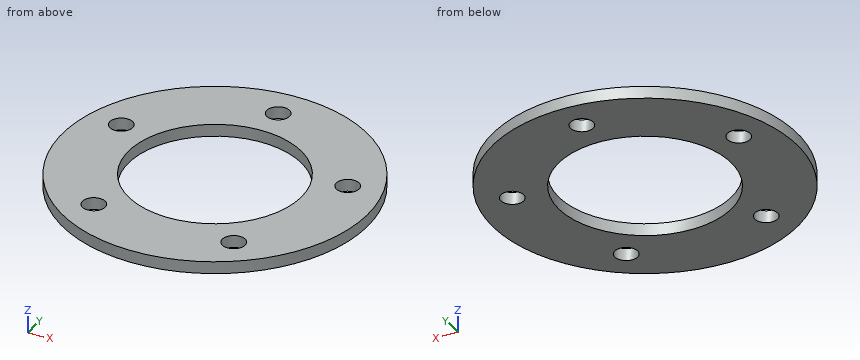
```python
from build123d import *

# Parameters (mm, degrees)
F0_R     = 38.1
F0_R_2   = 2.8575
F0_R_3   = 21.59
F1_DEPTH = 3.048


with BuildPart() as f1:
    # F0 (on Top) → F1 (new body)
    with BuildSketch(Plane.XY):
        Circle(F0_R)
        with Locations((-17.542451, -24.145112)):
            Circle(F0_R_2, mode=Mode.SUBTRACT)
        with Locations((17.542451, -24.145112)):
            Circle(F0_R_2, mode=Mode.SUBTRACT)
        with Locations((-28.384282, 9.222612)):
            Circle(F0_R_2, mode=Mode.SUBTRACT)
        Circle(F0_R_3, mode=Mode.SUBTRACT)
        with Locations((28.384282, 9.222612)):
            Circle(F0_R_2, mode=Mode.SUBTRACT)
        with Locations((0, 29.845)):
            Circle(F0_R_2, mode=Mode.SUBTRACT)
    extrude(amount=F1_DEPTH)


solid = f1.part
```
Read the model definition and answer for the solid it produces. Units are mm, in the model's axes. Coordinates: 2 decimals unless noted, no trailing zeros. Order: outer loops, then holes, each group sorted by start corner. A loop starts at its lowest first (then second) coordinate and runs counter-clockwise, first axis right, second up. Notation, with made-up numbers: (46.25, 30.25) - (72.25, 30.25) arc R13 cw to (72.25, 55.25) - close; hole circle Ø2 at (4, 56.25). An arc over 180 degrees is marked (long way). Answer as a JSON object with one key per item and string values. Group by question number.
Item 1: Consider probe 1 along Y at (x, z) = (0, 1.8); probe 2 along Y at (x, z) = (18.5, 2); probe 3 along X at (y, z) = (-25, 1.9). Determine where each line is inside the solid, lowest interval first. Write a range as from..to.
Item 2: Flat-ended cylindrical pins translate along their axes: P1, Ø6, axis at x = 15.5, y = -3.5, coming from the +Z side; P2, Ø7.5, axis at x = -28.38, y = 9.22, coming from the +Z side. Find the tip coordinate at first contact, or state that the pin passes through.
Item 3: Section D-D (x = 9.5) is taken. Give the vertices of the cut face in (y, z), plus the area to 3 significant figures.
Item 4: Section C-C (z = 2.05) is taken. Give the vertices of the cut face in (x, y) (1 decimal), plus the area to 3 significant figures.
Item 5: Section A-A (x = 0) is taken. Give the vertices of the cut face in (y, z).
Item 6: Section B-B (y = 0) is taken. Give the vertices of the cut face in (x, z), plus the area to 3 significant figures.
Results are:
{
 "1": {"probe 1": "y = -38.1..-21.59, 21.59..26.99, 32.7..38.1", "probe 2": "y = -33.31..-26.84, -21.45..-11.13, 11.13..33.31", "probe 3": "x = -28.75..-20.27, -14.82..14.82, 20.27..28.75"},
 "2": {"P1": "passes through", "P2": "stops at z = 3.05"},
 "3": {"outline": "(-36.9, 0) - (-19.39, 0) - (-19.39, 3.05) - (-36.9, 3.05) - close; (19.39, 0) - (36.9, 0) - (36.9, 3.05) - (19.39, 3.05) - close", "area": "107 mm^2"},
 "4": {"outline": "circle Ø76.2 at (0, 0); hole circle Ø5.7 at (-28.4, 9.2); hole circle Ø43.2 at (0, 0); hole circle Ø5.7 at (-17.5, -24.1); hole circle Ø5.7 at (0, 29.8); hole circle Ø5.7 at (17.5, -24.1); hole circle Ø5.7 at (28.4, 9.2)", "area": "2,970 mm^2"},
 "5": {"outline": "(-38.1, 0) - (-21.59, 0) - (-21.59, 3.05) - (-38.1, 3.05) - close; (21.59, 0) - (26.99, 0) - (26.99, 3.05) - (21.59, 3.05) - close; (32.7, 0) - (38.1, 0) - (38.1, 3.05) - (32.7, 3.05) - close"},
 "6": {"outline": "(-38.1, 0) - (-21.59, 0) - (-21.59, 3.05) - (-38.1, 3.05) - close; (21.59, 0) - (38.1, 0) - (38.1, 3.05) - (21.59, 3.05) - close", "area": "101 mm^2"}
}
